```python
from build123d import *

# Parameters (mm, degrees)
F0_W     = 11.887384
F0_H     = 40
F0_R     = 4.6
F1_DEPTH = 20
F0_R_2   = 2.7
F2_DEPTH = 10
F3_R     = 4.2
F4_DEPTH = 11.887384


with BuildPart() as f1:
    # F0 (on Top) → F1 (new body)
    with BuildSketch(Plane.XY):
        with Locations((-5.943692, -20)):
            Rectangle(F0_W, F0_H)
        with Locations((-5.943692, -32)):
            Circle(F0_R, mode=Mode.SUBTRACT)
        with Locations((-5.943692, -8)):
            Circle(F0_R, mode=Mode.SUBTRACT)
    extrude(amount=F1_DEPTH)

    # F0 (on Top) → F2 (join)
    with BuildSketch(Plane.XY):
        with Locations((-5.943692, -8)):
            Circle(F0_R)
        with Locations((-5.943692, -8)):
            Circle(F0_R_2, mode=Mode.SUBTRACT)
        with Locations((-5.943692, -32)):
            Circle(F0_R)
        with Locations((-5.943692, -32)):
            Circle(F0_R_2, mode=Mode.SUBTRACT)
    extrude(amount=F2_DEPTH)

    # F3 (on face) → F4 (cut, through all)
    with BuildSketch(Plane(origin=(-11.887384, 0, 0), x_dir=(0, -1, 0), z_dir=(-1, 0, 0))):
        with Locations((20, 10)):
            Circle(F3_R)
    extrude(amount=-F4_DEPTH, mode=Mode.SUBTRACT)


solid = f1.part
```
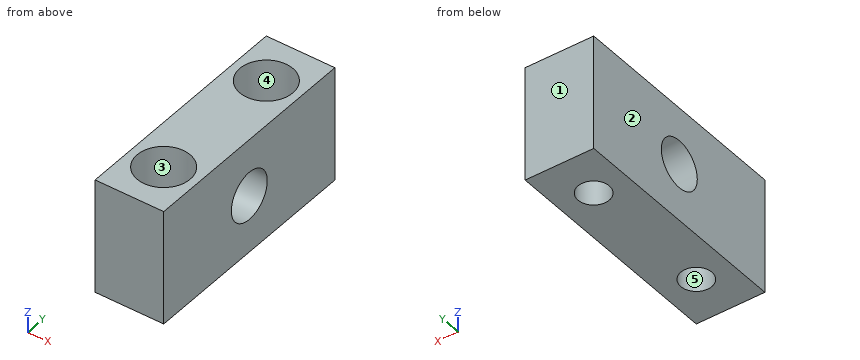
Part model, mm, in its own coordinate system. Face numbers are marked on the shaded views. A direction names the side the tool comes from. Give positions to 0.01 mm unless a question says otherwise; leave off trailing zeros. Write each loop counter-clockwise with the first axis right and the second up, starting at its lowest first coordinate (ties: lowest second). Pieces come first, ordered by that corner, then holes. Notation, with made-up numbers: (59, 81.5) -> (114, 81.5) arc R19 cw to (114, 112.5) -> close; hole circle Ø5 at (83, -26). An arc over 180 degrees is marked (long way). Put each result on its own line as item: value. Start each with the question number.
Item 1: Wall check: L1, parallel to Y at x = -6.75, z = 2.5; L2, parallel to Y at x = -6.5, z = 11.25; L3, parallel to Y at x = -5.5, z = 3.25. Give the ranges that are in metal, low to high. Write a range as [from, to].
Item 2: Pull direction Y, two halves, no side cores. Call the marked faces 1, 2 and 3: pulls with the +Y half, pulls with the -Y half, needs draft (parallel to the pull), parting line crosses it, or undercut.
Item 3: Pin check, flat tips, straight feed: pin 1 Ø3 at (x, y) = (-5.94, -32) entering from -Z; pin 2 Ø5.5 at (x, y) = (-5.94, -32) entering from +Z. Stop position of each tip, or through.
Item 4: Cut at B-B (z = 9.5). List the corners of the cut face in (x, y), then the cut area to 3 significant figures.
Item 5: Which spindle directions (+Z, -Z, +X, -X, +Y, -Y) get a long thin tool onto all of the face, cutting with end or side? Do the marked faces 4 and 5. Say none if no direction does.
Item 6: Cut at A-A (y = -32). List the corners of the cut face in (x, z).
Item 7: Cut at C-C (x = -9.25). List the corners of the cut face in (y, z), then the cut area to 3 significant figures.
Item 8: Cut at D-D (z = 3). List the corners of the cut face in (x, y).
Answer list:
1. L1: y = [-40, -34.58], [-29.42, -10.58], [-5.42, 0]
1. L2: y = [-40, -36.57], [-27.43, -24.01], [-15.99, -12.57], [-3.43, 0]
1. L3: y = [-40, -34.66], [-29.34, -10.66], [-5.34, 0]
2. face 1: pulls with the +Y half
2. face 2: needs draft
2. face 3: undercut
3. pin 1: passes through
3. pin 2: stops at z = 10
4. outline: (-11.89, -40) -> (0, -40) -> (0, -24.17) -> (-11.89, -24.17) -> close; (-11.89, -15.83) -> (0, -15.83) -> (0, 0) -> (-11.89, 0) -> close; hole circle Ø5.4 at (-5.94, -32); hole circle Ø5.4 at (-5.94, -8)
4. area: 331 mm2
5. face 4: +Z
5. face 5: +Z, -Z
6. outline: (-11.89, 0) -> (-8.64, 0) -> (-8.64, 10) -> (-10.54, 10) -> (-10.54, 20) -> (-11.89, 20) -> close; (-3.24, 0) -> (0, 0) -> (0, 20) -> (-1.34, 20) -> (-1.34, 10) -> (-3.24, 10) -> close
7. outline: (-40, 0) -> (0, 0) -> (0, 20) -> (-4.8, 20) -> (-4.8, 10) -> (-11.2, 10) -> (-11.2, 20) -> (-28.8, 20) -> (-28.8, 10) -> (-35.2, 10) -> (-35.2, 20) -> (-40, 20) -> close; hole circle Ø8.4 at (-20, 10)
7. area: 617 mm2
8. outline: (-11.89, -40) -> (0, -40) -> (0, 0) -> (-11.89, 0) -> close; hole circle Ø5.4 at (-5.94, -32); hole circle Ø5.4 at (-5.94, -8)
